Could you check a few things on this model? Use its own coordinates, in mm. A direction names the side the tool comes from. Give positions to 0.01 mm unless a question says otherwise; leave off trailing zeros. Write each loop counter-clockwise with the first axis right and the second up, starting at its lowest first coordinate (ties: lowest second). Pieces come first, ordered by that corner, then holes. Notation, with made-up numbers: (-32.75, 84) - (19.25, 84) arc R27 cw to (19.25, 110) - close; hole circle Ø9 at (-28, 87.5). An arc over 180 degrees is marked (long way). Answer in a Markdown table with one row per item.
from build123d import *

# Parameters (mm, degrees)
SKETCH_1_R      = 1.625
SKETCH_1_W      = 5
SKETCH_1_H      = 3
EXTRUDE_1_DEPTH = 3
CHAMFER_1_SIZE  = 0.5
FILLET_1_R      = 1
FILLET_2_R      = 0.5
EXTRUDE_2_DEPTH = 3


with BuildPart() as part:
    # 草图1 → 凸台-拉伸1 (new body)
    with BuildSketch(Plane(origin=(1.5, 0, 0), x_dir=(0, 0, -1), z_dir=(1, 0, 0))):
        with BuildLine():
            Line((-7.154542269, -8.576560818), (1.041442411, -7.427341227))
            ThreePointArc((1.041442411, -7.427341227), (6.705040976, -3.360420437), (6.573553871, 3.610871017))
            Line((6.573553871, 3.610871017), (2.332034096, 11.332514521))
            ThreePointArc((2.332034096, 11.332514521), (2.051803428, 11.696549741), (1.674538126, 11.958698097))
            Line((1.674538126, 11.958698097), (-3.312005463, 14.389232718))
            ThreePointArc((-3.312005463, 14.389232718), (-3.689270765, 14.651381075), (-3.969501433, 15.015416295))
            Line((-3.969501433, 15.015416295), (-8.120214479, 22.571747074))
            ThreePointArc((-8.120214479, 22.571747074), (-8.297319992, 23.137447109), (-8.241448295, 23.727583743))
            Line((-8.241448295, 23.727583743), (-7.088083158, 27.546610192))
            ThreePointArc((-7.088083158, 27.546610192), (-7.032211461, 28.136746826), (-7.209316974, 28.702446861))
            Line((-7.209316974, 28.702446861), (-10.617630753, 34.907247345))
            ThreePointArc((-10.617630753, 34.907247345), (-16.500374515, 37.269578211), (-19.97127937, 31.964853827))
            ThreePointArc((-19.97127937, 31.964853827), (-19.942635933, 31.401924032), (-19.977533596, 30.839347323))
            Line((-19.977533596, 30.839347323), (-21.975677109, 14.034639668))
            ThreePointArc((-21.975677109, 14.034639668), (-23.620446364, 10.886564387), (-26.940702253, 9.625))
            Line((-26.940702253, 9.625), (-29.188611699, 9.625))
            ThreePointArc((-29.188611699, 9.625), (-29.989522914, 9.560437288), (-30.769750529, 9.36841649))
            Line((-30.769750529, 9.36841649), (-36.474341649, 7.466886117))
            ThreePointArc((-36.474341649, 7.466886117), (-37.216863278, 6.920926597), (-37.5, 6.04386117))
            Line((-37.5, 6.04386117), (-37.5, 4.625))
            Line((-37.5, 4.625), (-32.5, 4.625))
            Line((-32.5, 4.625), (-32.5, 1.625))
            Line((-32.5, 1.625), (-27.5, 1.625))
            Line((-27.5, 1.625), (-27.5, -1.625))
            Line((-27.5, -1.625), (-32.5, -1.625))
            Line((-32.5, -1.625), (-32.5, -4.625))
            Line((-32.5, -4.625), (-37.5, -4.625))
            Line((-37.5, -4.625), (-37.5, -5.609450558))
            ThreePointArc((-37.5, -5.609450558), (-37.242100846, -6.450393772), (-36.557086015, -7.002165594))
            Line((-36.557086015, -7.002165594), (-33.394041364, -8.267383454))
            ThreePointArc((-33.394041364, -8.267383454), (-32.482625588, -8.534781934), (-31.537087982, -8.625))
            Line((-31.537087982, -8.625), (-7.848837209, -8.625))
            ThreePointArc((-7.848837209, -8.625), (-7.500845895, -8.612875504), (-7.154542269, -8.576560818))
        make_face()
        with Locations(Location((-15, 32.5, 0), (0, 0, 180))):
            Circle(SKETCH_1_R, mode=Mode.SUBTRACT)
        with Locations(Location((0, 0, 0), (0, 0, 180))):
            Circle(SKETCH_1_R, mode=Mode.SUBTRACT)
        with Locations((-22, 3.125)):
            Rectangle(SKETCH_1_W, SKETCH_1_H, mode=Mode.SUBTRACT)
        with Locations((-22, -3.125)):
            Rectangle(SKETCH_1_W, SKETCH_1_H, mode=Mode.SUBTRACT)
        with BuildLine():
            Line((-9.961966793, 5.476712688), (-17.295484898, 21.366001917))
            ThreePointArc((-17.295484898, 21.366001917), (-16.439907786, 23.68828265), (-14.117627052, 22.832705538))
            Line((-14.117627052, 22.832705538), (-6.784108947, 6.943416309))
            ThreePointArc((-6.784108947, 6.943416309), (-7.639686059, 4.621135575), (-9.961966793, 5.476712688))
        make_face(mode=Mode.SUBTRACT)
    extrude(amount=-EXTRUDE_1_DEPTH)

    # 倒角1
    chamfer_1_edges = [part.edges().sort_by_distance(p)[0] for p in [
        (-1.5, 0, 27.5),
        (-1.5, -3.125, 24.5),
        (-1.5, -1.625, 22),
        (-1.5, -3.125, 19.5),
        (-1.5, -4.625, 22),
        (1.5, -3.125, 24.5),
        (1.5, -4.625, 22),
        (1.5, -3.125, 19.5),
        (-1.5, -1.625, 30),
        (1.5, -1.625, 22),
        (-1.5, -3.125, 32.5),
        (-1.5, -4.625, 35),
        (-1.5, 4.621135575, 7.639686059),
        (-1.5, 13.421357302, 13.628725845),
        (-1.5, 23.68828265, 16.439907786),
        (-1.5, 14.888060923, 10.450868),
        (-1.5, -5.117225279, 37.5),
        (1.5, 4.621135575, 7.639686059),
        (1.5, 14.888060923, 10.450868),
        (1.5, 23.68828265, 16.439907786),
        (1.5, 13.421357302, 13.628725845),
        (-1.5, -6.450393772, 37.242100846),
        (-1.5, -7.634774524, 34.975563689),
        (-1.5, -8.534781934, 32.482625588),
        (-1.5, -3.360420437, -6.705040976),
        (-1.5, -8.625, 19.692962596),
        (-1.5, 7.471692769, -4.452793984),
        (-1.5, 11.696549741, -2.051803428),
        (-1.5, 13.173965408, 0.818733668),
        (-1.5, 14.651381075, 3.689270765),
        (1.5, -8.625, 19.692962596),
        (1.5, -8.534781934, 32.482625588),
        (1.5, -7.634774524, 34.975563689),
        (1.5, -6.450393772, 37.242100846),
        (1.5, -5.117225279, 37.5),
        (-1.5, 18.793581684, 6.044857956),
        (1.5, -4.625, 35),
        (1.5, -3.125, 32.5),
        (1.5, -1.625, 30),
        (1.5, 0, 27.5),
        (1.5, 1.625, 30),
        (1.5, 3.125, 32.5),
        (1.5, 4.625, 35),
        (1.5, 5.334430585, 37.5),
        (1.5, 6.920926597, 37.216863278),
        (1.5, 8.417651304, 33.622046089),
        (-1.5, 23.137447109, 8.297319992),
        (1.5, 9.560437288, 29.989522914),
        (1.5, 9.625, 28.064656976),
        (1.5, 10.886564387, 23.620446364),
        (1.5, 22.436993496, 20.976605353),
        (1.5, 31.401924032, 19.942635933),
        (1.5, 37.269578211, 16.500374515),
        (1.5, 31.804847103, 8.913473863),
        (1.5, 28.136746826, 7.032211461),
        (1.5, 25.637096968, 7.664765726),
        (1.5, 23.137447109, 8.297319992),
        (-1.5, 25.637096968, 7.664765726),
        (1.5, 18.793581684, 6.044857956),
        (1.5, 14.651381075, 3.689270765),
        (1.5, 13.173965408, 0.818733668),
        (1.5, 11.696549741, -2.051803428),
        (1.5, 7.471692769, -4.452793984),
        (1.5, -3.360420437, -6.705040976),
        (1.5, -8.001951023, 3.056549929),
        (1.5, -8.612875504, 7.500845895),
        (-1.5, 28.136746826, 7.032211461),
        (-1.5, 31.804847103, 8.913473863),
        (-1.5, -8.612875504, 7.500845895),
        (-1.5, 37.269578211, 16.500374515),
        (-1.5, 31.401924032, 19.942635933),
        (-1.5, 22.436993496, 20.976605353),
        (-1.5, 10.886564387, 23.620446364),
        (-1.5, 9.625, 28.064656976),
        (-1.5, 9.560437288, 29.989522914),
        (-1.5, 8.417651304, 33.622046089),
        (-1.5, 32.5, 13.375),
        (1.5, 32.5, 13.375),
        (-1.5, 6.920926597, 37.216863278),
        (-1.5, 0, -1.625),
        (1.5, 0, -1.625),
        (-1.5, 5.334430585, 37.5),
        (-1.5, 4.625, 35),
        (-1.5, 3.125, 19.5),
        (-1.5, -8.001951023, 3.056549929),
        (-1.5, 1.625, 22),
        (-1.5, 3.125, 24.5),
        (-1.5, 4.625, 22),
        (1.5, 3.125, 19.5),
        (1.5, 4.625, 22),
        (1.5, 3.125, 24.5),
        (1.5, 1.625, 22),
        (-1.5, 3.125, 32.5),
        (-1.5, 1.625, 30),
    ]]
    chamfer(chamfer_1_edges, length=CHAMFER_1_SIZE)

    # 圆角1
    # the kernel refuses this fillet: 1 mm, written as the material it takes off along each edge
    with BuildSketch(Plane(origin=(3.577747849, -4.625, 37.5), x_dir=(0, -0.9999997524396673, -0.000703648068189184), z_dir=(-1, 0, 0))) as fillet_1_piece_1:
        with BuildLine():
            CenterArc((1.000703571, -0.999537948), FILLET_1_R, 88.258193912, 91.782122156)
            Line((0.000703818, -1.000241596), (-0.099296157, -1.000311961))
            Line((-0.099296157, -1.000311961), (-0.099999975, -7.0365e-05))
            Line((-0.099999975, -7.0365e-05), (-7.0365e-05, 0.099999975))
            ThreePointArc((-7.0365e-05, 0.099999975), (0.984379949, 0.100692682), (1.034138696, 0.099953795))
            Line((1.034138696, 0.099953795), (1.03109914, 0))
        make_face()
    extrude(amount=7.155495698, mode=Mode.SUBTRACT)
    with BuildSketch(Plane(origin=(3.5, 4.625, 37.5), x_dir=(0, 0, -1), z_dir=(-1, 0, 0))) as fillet_1_piece_2:
        with BuildLine():
            CenterArc((FILLET_1_R, -FILLET_1_R), FILLET_1_R, 90, 90)
            Line((0, -FILLET_1_R), (0, 0))
            Line((0, 0), (FILLET_1_R, 0))
        make_face()
    extrude(amount=7, mode=Mode.SUBTRACT)

    # 圆角2
    fillet_2_edges = [part.edges().sort_by_distance(p)[0] for p in [
        (0, 1.625, 32.5),
        (0, -1.625, 32.5),
    ]]
    fillet(fillet_2_edges, radius=FILLET_2_R)

    # Sketch 3D_1 → 凸台-拉伸2 (add)
    with BuildSketch(Plane(origin=(1.5, 22.89191641, 19.156270075), x_dir=(0, -0.8525521578237779, -0.5226421511799639), z_dir=(1, 0, 0))):
        Polygon((0, 0), (16.191873752, -5.770917197), (27.468575768, 0), (19.557121084, 8.11942404), (6.27778787, 5.658813531), (-1.099641064, 7.65553458), (-1.226258679, 2.829349925), align=None)
    extrude(amount=-EXTRUDE_2_DEPTH)


solid = part.part
1) Imagine slicing it at B-B (z = 0). List the corners of the cut face in (x, y) for me (3 decimals), then the cut area to 3 significant figures.
Check values:
| item | result |
|---|---|
| outline | (-1.5, -7.068) - (-1, -7.573) - (1, -7.573) - (1.5, -7.068) - (1.5, -2.125) - (1, -1.625) - (-1, -1.625) - (-1.5, -2.125) - close; (-1.5, 2.125) - (-1, 1.625) - (1, 1.625) - (1.5, 2.125) - (1.5, 12.219) - (1, 12.775) - (-1, 12.775) - (-1.5, 12.219) - close |
| area | 50.3 mm2 |
2) On a 3-axis mill with a long thin cutter (end or side, diameter ignored), from which of +Z, -Z, +X, -X, +Y, -Y can I reach the whole of each face in a straight line? I mean faces 4 (the face through (-1.254, 18.619, 6.238)), 5 (the face through (0, 1.625, 22)), 6 (the face through (0.014, 18.741, 6.016)). Say none if no direction works.
Check values:
| item | result |
|---|---|
| face 4 | -Z, -X |
| face 5 | +X, -X |
| face 6 | -Z, +X, -X |
3) Imagine slicing it at A-A (z = 15). List the corners of the cut face in (x, y) for me (3 decimals).
Check values:
| item | result |
|---|---|
| outline | (-1.5, -8.125) - (-1, -8.625) - (1, -8.625) - (1.5, -8.125) - (1.5, 30.375) - (1, 30.875) - (-1, 30.875) - (-1.5, 30.375) - close; (-1.5, 34.625) - (-1, 34.125) - (1, 34.125) - (1.5, 34.625) - (1.5, 37) - (1, 37.5) - (-1, 37.5) - (-1.5, 37) - close |
4) Will these pins go through, and if not, where does the flat tip stop? P1, Ø0.6, axis at x = 0, z = 35, coming from the +Y side; P2, Ø1, axis at x = 0, y = 3, coming from the +Z side; P3, Ø1.6, axis at x = 0.5, z = 30, coming from the +Y side (3 decimals).
Check values:
| item | result |
|---|---|
| P1 | stops at y = 8.06 |
| P2 | stops at z = 32.5 |
| P3 | stops at y = 9.625 |
5) If I drill on line 1 (Y direction, x = 0.5, z = 15) (3 decimals); line 2 (Z direction, x = -0.2, y = -1); line 3 (Y direction, x = -0.05, z = 30) (3 decimals), over which ranges is the centre line in solid material (lowest first)?
Check values:
| item | result |
|---|---|
| line 1 | y = -8.625 to 30.875, 34.125 to 37.5 |
| line 2 | z = -7.43 to -1.28, 1.28 to 27.5 |
| line 3 | y = -8.625 to -1.625, 1.625 to 9.559 |
6) Imagine slicing it at C-C (z = 5). List the corners of the cut face in (x, y) for me.
Check values:
| item | result |
|---|---|
| outline | (-1.5, -7.77) - (-1, -8.27) - (1, -8.27) - (1.5, -7.77) - (1.5, 15.85) - (1, 16.89) - (-1, 16.89) - (-1.5, 15.85) - close |
7) We'd pull the mould along Y, two halves only. Please class faces 1 (the face through (-1.254, 8.19, 33.502)), 2 (the face through (0.014, 25.61, 7.673)), 3 (the face through (-1.254, -7.391, 34.904)): +Y half, -Y half, draft (parallel to the pull), parting line (faces both ways), or undercut.
Check values:
| item | result |
|---|---|
| face 1 | +Y half |
| face 2 | undercut |
| face 3 | -Y half |
